```python
from build123d import *

# Parameters (mm, degrees)
SKETCH1_W              = 43
SKETCH1_H              = 112
SKETCH1_R              = 1.5
BOARD_DEPTH            = 2
SKETCH2_W              = 16
SKETCH2_H              = 40
SKETCH2_W_2            = 6
SKETCH2_H_2            = 10
F_7SEG_DEPTH           = 11
SKETCH3_W              = 10
SKETCH3_H              = 20
SKETCH3_H_2            = 10
IC_DEPTH               = 8
SKETCH5_W              = 9
SKETCH5_H              = 17
BIENTROA_DEPTH         = 23
SKETCH6_R              = 3.4
BIENTROB_DEPTH         = 15
SKETCH7_W              = 10
SKETCH7_H              = 5
IRF540_DEPTH           = 26
SKETCH8_W              = 17
SKETCH8_H              = 10
DOMINO_DEPTH           = 10
SKETCH9_W              = 22
SKETCH9_H              = 30
EXTRUDE_7805_DEPTH     = 30
SPLIT2_SURFACE_1_BACK  = 131.572
SPLIT2_SURFACE_1_DEPTH = 263.144
SPLIT2_SURFACE_2_BACK  = 131.572
SPLIT2_SURFACE_2_DEPTH = 263.144


with BuildPart() as part:
    # Sketch1 → Board (new body)
    with BuildSketch(Plane(origin=(0, 0, 0), x_dir=(1, 0, 0), z_dir=(0, 1, 0))):
        Rectangle(SKETCH1_W, SKETCH1_H)
        with Locations(Location((18.1, -52.6, 0), (0, 0, 270))):
            Circle(SKETCH1_R, mode=Mode.SUBTRACT)
        with Locations(Location((-16.5, 52, 0), (0, 0, 270))):
            Circle(SKETCH1_R, mode=Mode.SUBTRACT)
        with Locations(Location((-18.1, 7, 0), (0, 0, 270))):
            Circle(SKETCH1_R, mode=Mode.SUBTRACT)
    extrude(amount=BOARD_DEPTH)

    # Sketch2 → 7SEG (add)
    with BuildSketch(Plane(origin=(0, 2, 0), x_dir=(1, 0, 0), z_dir=(0, 1, 0))):
        with Locations((8.5, 31)):
            Rectangle(SKETCH2_W, SKETCH2_H)
        with Locations((12.5, 5)):
            Rectangle(SKETCH2_W_2, SKETCH2_H_2)
    extrude(amount=F_7SEG_DEPTH)

    # Sketch3 → IC (add)
    with BuildSketch(Plane(origin=(0, 2, 0), x_dir=(1, 0, 0), z_dir=(0, 1, 0))):
        with Locations((-6.5, 26)):
            Rectangle(SKETCH3_W, SKETCH3_H)
        with Locations((-0.5, 5)):
            Rectangle(SKETCH3_W, SKETCH3_H_2)
        with Locations((-0.5, -17)):
            Rectangle(SKETCH3_W, SKETCH3_H_2)
    extrude(amount=IC_DEPTH)

    # Sketch5 → BienTroA (add)
    with BuildSketch(Plane(origin=(0, 2, 0), x_dir=(1, 0, 0), z_dir=(0, 1, 0))):
        with Locations((11, -14.5)):
            Rectangle(SKETCH5_W, SKETCH5_H)
    extrude(amount=BIENTROA_DEPTH)

    # Sketch6 → BienTroB (add)
    with BuildSketch(Plane(origin=(15.5, 0, 0), x_dir=(0, 0, -1), z_dir=(1, 0, 0))):
        with Locations(Location((-14.5, 16.6, 0), (0, 0, 180))):
            Circle(SKETCH6_R)
    extrude(amount=BIENTROB_DEPTH)

    # Sketch7 → IRF540 (add)
    with BuildSketch(Plane(origin=(0, 2, 0), x_dir=(1, 0, 0), z_dir=(0, 1, 0))):
        with Locations((9.5, -47.5)):
            Rectangle(SKETCH7_W, SKETCH7_H)
    extrude(amount=IRF540_DEPTH)

    # Sketch8 → Domino (add)
    with BuildSketch(Plane(origin=(0, 2, 0), x_dir=(1, 0, 0), z_dir=(0, 1, 0))):
        with Locations((-7, -50)):
            Rectangle(SKETCH8_W, SKETCH8_H)
    extrude(amount=DOMINO_DEPTH)

    # Sketch9 → 7805 (add)
    with BuildSketch(Plane(origin=(0, 2, 0), x_dir=(1, 0, 0), z_dir=(0, 1, 0))):
        with Locations((-17.5, -26)):
            Rectangle(SKETCH9_W, SKETCH9_H)
    extrude(amount=EXTRUDE_7805_DEPTH)


with BuildPart() as body_2:
    # Split2: the piece behind the surface
    add(part.part)
    # Split2 surface: a surface, the sketch's curves swept straight by 263.144 mm
    with BuildLine(Plane(origin=(0, 2, 0), x_dir=(1, 0, 0), z_dir=(0, 1, 0)).offset(-SPLIT2_SURFACE_1_BACK), mode=Mode.PRIVATE) as split2_surface_1_path:
        Line((21.5, 11), (-21.5, 11))
    split2_surface_1 = Shell.extrude(split2_surface_1_path.wire(), (0 * SPLIT2_SURFACE_1_DEPTH, 1 * SPLIT2_SURFACE_1_DEPTH, 0 * SPLIT2_SURFACE_1_DEPTH))
    split(bisect_by=split2_surface_1, keep=Keep.BOTTOM)


with BuildPart() as part_1:
    add(part.part)

    # Split2: split by a surface, the side it looks to stays
    # Split2 surface: a surface, the sketch's curves swept straight by 263.144 mm
    with BuildLine(Plane(origin=(0, 2, 0), x_dir=(1, 0, 0), z_dir=(0, 1, 0)).offset(-SPLIT2_SURFACE_2_BACK), mode=Mode.PRIVATE) as split2_surface_2_path:
        Line((21.5, 11), (-21.5, 11))
    split2_surface_2 = Shell.extrude(split2_surface_2_path.wire(), (0 * SPLIT2_SURFACE_2_DEPTH, 1 * SPLIT2_SURFACE_2_DEPTH, 0 * SPLIT2_SURFACE_2_DEPTH))
    split(bisect_by=split2_surface_2, keep=Keep.TOP)


solid = part_1.part
```
CAD build for the part. Positions are in the model's coordinates, mm. A direction names the side the tool comes from. Coordinates: 2 decimals unless noted, no trailing zeros. Write each loop counter-clockwise with the first axis right and the second up, starting at its lowest first coordinate (ties: lowest second). Pieces come first, ordered by that corner, then holes.
(1) Cut at A-A, the plane y = 16.6. List the corners of the cut face in (x, z), and give its area (3 significant figures).
(2) Flat gauge pins, fed straight in: pin 1 (12 mm diameter, centred on x = 5, y = 10, fed in from +Z); pin 2 (1.5 mm diameter, centred on x = -2, z = 32, fed in from +Y); pin 3 (5 mm diameter, centred on x = -11, z = 50.5, fed in from +Y); pin 4 (1.5 mm diameter, centred on x = -6, z = 11, fed in from +Y). Where does each tip first touch, or does it go through?
(3) Two-plate mould, pull along X, no slides. Class faces 6 (the face through (-18, 17, 41)), 7 (the face through (4.5, 6, -5)), 8 (the face through (21.5, 1, 23)): +X half, -X half, draft (parallel to the pull), parting line (faces both ways), or undercut.
(4) 3-axis set-ups, long thin cutter, end or side, ignore diameter. For faces 1 (the face through (4.5, 15, 48)), 2 (the face through (9.5, 7, -5)), 3 (the face through (-21.5, 1, 23)), 4 (the face through (15.5, 7, -5)), 5 (the face through (-1, 6, 0)): which of +Z, -Z, +X, -X, +Y, -Y reach the whole face in a straight line?
(5) Drill centre lines: probe 1 along Z at (x, y) = (13.5, 4); probe 2 along X at (y, z) = (1, -7); probe 3 along Z at (x, y) = (0, 9). Where is each one in solid material? Low to high.
(6) Cut at D-D, the plane y = 5. List the corners of the cut face in (x, z).
(7) Cut at C-C, the plane y = 27. List the corners of the cut face in (x, z), and give its area (3 significant figures).
(8) Cut at B-B, the plane z = -7. List the corners of the cut face in (x, y), and give its area (3 significant figures).
Geometry says:
1. outline: (-28.5, 11) - (-6.5, 11) - (-6.5, 41) - (-28.5, 41) - close; (4.5, 45) - (14.5, 45) - (14.5, 50) - (4.5, 50) - close; (6.5, 6) - (15.5, 6) - (15.5, 11.1) - (30.5, 11.1) - (30.5, 17.9) - (15.5, 17.9) - (15.5, 23) - (6.5, 23) - close
1. area: 965 mm2
2. pin 1: stops at z = 55
2. pin 2: stops at y = 2
2. pin 3: stops at y = 12
2. pin 4: stops at y = 32
3. face 6: draft
3. face 7: undercut
3. face 8: +X half
4. face 1: +Z, +Y
4. face 2: -Z, +Y
4. face 3: +Z, -Z, -X, -Y
4. face 4: +Z, -Z, +X, +Y
4. face 5: +X, -X, +Y
5. probe 1: z = -10 to 0, 6 to 23, 45 to 50
5. probe 2: x = -21.5 to -19.6, -16.6 to 21.5
5. probe 3: z = -10 to 0, 12 to 22, 45 to 55
6. outline: (-28.5, 11) - (-6.5, 11) - (-6.5, 41) - (-28.5, 41) - close; (-15.5, 45) - (1.5, 45) - (1.5, 55) - (-15.5, 55) - close; (-5.5, -10) - (4.5, -10) - (4.5, 0) - (-5.5, 0) - close; (-5.5, 12) - (4.5, 12) - (4.5, 22) - (-5.5, 22) - close; (4.5, 45) - (14.5, 45) - (14.5, 50) - (4.5, 50) - close; (6.5, 6) - (15.5, 6) - (15.5, 23) - (6.5, 23) - close; (9.5, -10) - (15.5, -10) - (15.5, 0) - (9.5, 0) - close
7. outline: (-28.5, 11) - (-6.5, 11) - (-6.5, 41) - (-28.5, 41) - close; (4.5, 45) - (14.5, 45) - (14.5, 50) - (4.5, 50) - close
7. area: 710 mm2
8. outline: (-21.5, 0) - (-19.6, 0) - (-19.6, 2) - (-21.5, 2) - close; (-16.6, 0) - (21.5, 0) - (21.5, 2) - (15.5, 2) - (15.5, 13) - (9.5, 13) - (9.5, 2) - (4.5, 2) - (4.5, 10) - (-5.5, 10) - (-5.5, 2) - (-16.6, 2) - close
8. area: 226 mm2
